Answer from the drawing. Dimensions are ordinates in mm from the lowest x, y and z of the part. Coordinates: 2 decimals unless noted, no trailing zeros. Write each loop counter-clockwise with the first axis right and the second up, starting at its lowest first coordinate (ties: lowest second). Pieces come first, ordered by that corner, then holes. Notation, with made-up numbers: (2.5, 76.5) -> (53.5, 76.5) arc R15 ccw to (53.5, 101.5) -> close; hole circle Ø2 at (15.25, 36). An arc over 180 degrees is marked (long way). Return JSON: item names as keys, results as strings.
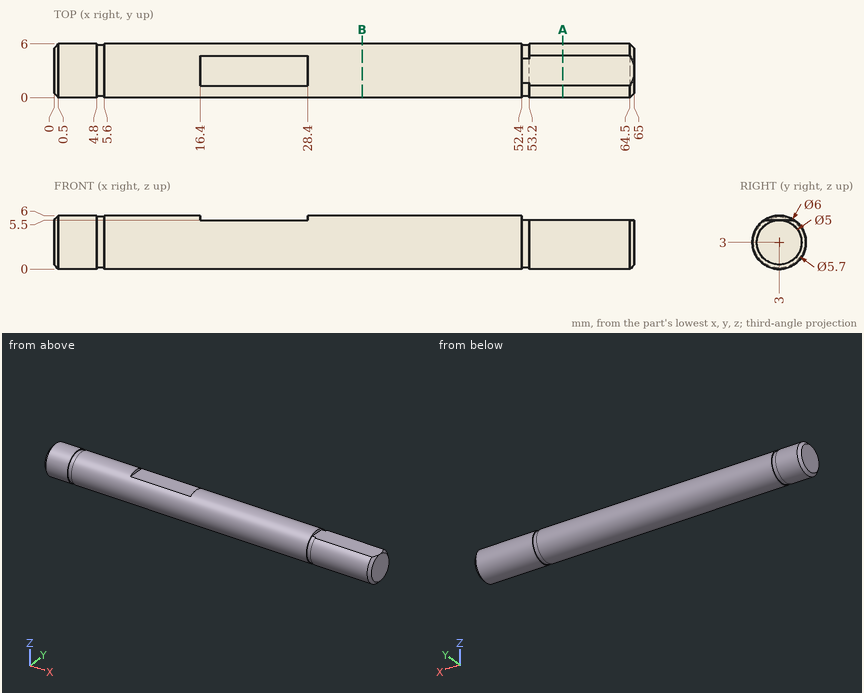
1. The part is cut by section A-A (x = 57). Determine the outline of the cut face in (y, z).
Taken from the geometry:
{"outline": "(1.34, 5.5) arc R3 ccw (long way) to (4.66, 5.5) -> close"}
2. The part is cut by section B-B (x = 34.5). Determine the outline of the cut face in (y, z).
Taken from the geometry:
{"outline": "circle Ø6 at (3, 3)"}
3. Flat-ended cylindrical pins translate along their axes: pin 1 Ø3.5 at (x, y) = (22, 3) entering from +Z; pin 2 Ø1.5 at (x, y) = (38.5, 4.5) entering from +Z. Find the tip coordinate at first contact, or state that the pin passes through.
Taken from the geometry:
{"pin 1": "stops at z = 5.5", "pin 2": "stops at z = 5.9"}
4. Consider L1, parallel to X at y = 0.6, z = 4.75; L2, parallel to X at y = 5.75, z = 4; L3, parallel to Z at x = 12.5, y = 3.9. Determine where each line is inside the solid, lowest interval first.
Taken from the geometry:
{"L1": "x = 0.47 to 4.8, 5.6 to 52.4, 53.2 to 64.53", "L2": "x = 0.43 to 4.8, 5.6 to 52.4, 53.2 to 64.57", "L3": "z = 0.14 to 5.86"}
